Check sheet for the modelled part. Datum: model origin and axes. Units: mm. A direction names the side the tool comes from. Round coordinates to 2 decimals unless told otherwise and drop trailing zeros. Order: outer loops, then holes, each group sorted by start corner. A loop starts at its lowest first (then second) coordinate and runs counter-clockwise, first axis right, second up.
Autodesk Inventor part; units mm, degrees
ref_plane "a1_XY" through (0, 8.636, -14.224) normal (0, 1, 0) x (1, 0, 0)
ref_plane "a1_YZ" through (0, 8.636, -14.224) normal (1, 0, 0) x (0, 0, -1)
ref_plane "a1_ZX" through (0, 8.636, -14.224) normal (0, 0, -1) x (0, 1, 0)
sketch "Sketch_1" plane through (0, 0, 0) normal (0, 0, 1) x (1, 0, 0)
  line L0 (0, 0) -> (0, 8.636)
  line L1 (0, 8.636) -> (14.224, 8.636)
  line L2 (14.224, 8.636) -> (14.224, 0)
  line L3 (14.224, 0) -> (0, 0)
  line L4 (0, 0) -> (0, 8.636)
revolve "Revolution1" add sketch "Sketch_1" angle 360 about axis through (0, 0, 0) along (0, -1, 0)
sketch "Sketch_37" plane through (0, 0, 0) normal (0, 0, 1) x (1, 0, 0)
  line L0 (-5.9667, 5.08) -> (-14.224, 5.08)
  line L1 (-14.224, 5.08) -> (-14.224, 9.0488)
  line L2 (-14.224, 9.0488) -> (-13.716, 9.0488)
  line L3 (-13.716, 9.0488) -> (-13.716, 7.493)
  line L4 (-13.716, 7.493) -> (-13.2867, 7.0637)
  line L5 (-13.2867, 7.0637) -> (-7.112, 7.0637)
  line L6 (-7.112, 7.0637) -> (-5.9667, 5.08)
  line L7 (-5.9667, 5.08) -> (-14.224, 5.08)
revolve "Revolution2" cut sketch "Sketch_37" angle 360 about axis through (-5.9667, 5.08, 0) along (1, 0, 0)
thread "Thread1"
sketch "Sketch3" plane through (0, 0, 0) normal (0, -1, 0) x (1, 0, 0)
  point P0 (0, 0)
hole "Hole1" at (0, 0, 0) direction (0, 1, 0) diameter 15.494 depth 2.54
sketch "Sketch4" plane through (0, 8.636, 0) normal (0, 1, 0) x (1, 0, 0)
  point P0 (0, -11.176)
hole "Hole2" at (0, 8.636, 11.176) direction (0, -1, 0) diameter 3.048 depth 8.636 counterbore diameter 4.7752 counterbore depth 3.048
sketch "Sketch5" plane through (0, 8.636, 0) normal (0, 1, 0) x (1, 0, 0)
  point P0 (0, 11.176)
hole "Hole3" at (0, 8.636, -11.176) direction (0, -1, 0) diameter 3.048 depth 8.636 counterbore diameter 4.7752 counterbore depth 3.048
sketch "Sketch6" plane through (0, 0, 0) normal (0, -1, 0) x (1, 0, 0)
  point P0 (-7.9026, 7.9026)
hole "Hole4" at (-7.9026, 0, 7.9026) direction (0, 1, 0) diameter 3.048 depth 2.54
sketch "Sketch7" plane through (0, 0, 0) normal (0, -1, 0) x (1, 0, 0)
  point P0 (7.9026, 7.9026)
hole "Hole5" at (7.9026, 0, 7.9026) direction (0, 1, 0) diameter 3.048 depth 2.54
sketch "Sketch8" plane through (0, 0, 0) normal (0, -1, 0) x (1, 0, 0)
  point P0 (7.9026, -7.9026)
hole "Hole6" at (7.9026, 0, -7.9026) direction (0, 1, 0) diameter 3.048 depth 2.54
sketch "Sketch9" plane through (0, 0, 0) normal (0, -1, 0) x (1, 0, 0)
  point P0 (-7.9026, -7.9026)
hole "Hole7" at (-7.9026, 0, -7.9026) direction (0, 1, 0) diameter 3.048 depth 2.54
ref_plane "a1_XY" through (0, 8.636, -14.224) normal (0, 1, 0) x (1, 0, 0)
ref_plane "a1_YZ" through (0, 8.636, -14.224) normal (1, 0, 0) x (0, 0, -1)
ref_plane "a1_ZX" through (0, 8.636, -14.224) normal (0, 0, -1) x (0, 1, 0)
ref_plane "a2_XY" through (0, 8.636, 14.224) normal (0, 1, 0) x (1, 0, 0)
ref_plane "a2_YZ" through (0, 8.636, 14.224) normal (1, 0, 0) x (0, 0, -1)
ref_plane "a2_ZX" through (0, 8.636, 14.224) normal (0, 0, -1) x (0, 1, 0)
ref_plane "ar3_XY" through (-7.9026, 2.54, 7.9026) normal (0, 1, 0) x (1, 0, 0)
ref_plane "ar3_YZ" through (-7.9026, 2.54, 7.9026) normal (1, 0, 0) x (0, 0, -1)
ref_plane "ar3_ZX" through (-7.9026, 2.54, 7.9026) normal (0, 0, -1) x (0, 1, 0)
ref_plane "ar4_XY" through (7.9026, 2.54, 7.9026) normal (0, 1, 0) x (1, 0, 0)
ref_plane "ar4_YZ" through (7.9026, 2.54, 7.9026) normal (1, 0, 0) x (0, 0, -1)
ref_plane "ar4_ZX" through (7.9026, 2.54, 7.9026) normal (0, 0, -1) x (0, 1, 0)
ref_plane "ar5_XY" through (7.9026, 2.54, -7.9026) normal (0, 1, 0) x (1, 0, 0)
ref_plane "ar5_YZ" through (7.9026, 2.54, -7.9026) normal (1, 0, 0) x (0, 0, -1)
ref_plane "ar5_ZX" through (7.9026, 2.54, -7.9026) normal (0, 0, -1) x (0, 1, 0)
ref_plane "ar6_XY" through (-7.9026, 2.54, -7.9026) normal (0, 1, 0) x (1, 0, 0)
ref_plane "ar6_YZ" through (-7.9026, 2.54, -7.9026) normal (1, 0, 0) x (0, 0, -1)
ref_plane "ar6_ZX" through (-7.9026, 2.54, -7.9026) normal (0, 0, -1) x (0, 1, 0)
ref_plane "b1_XY" through (0, 8.636, 0) normal (0, 1, 0) x (1, 0, 0)
ref_plane "b1_YZ" through (0, 8.636, 0) normal (1, 0, 0) x (0, 0, -1)
ref_plane "b1_ZX" through (0, 8.636, 0) normal (0, 0, -1) x (0, 1, 0)
ref_plane "c1_XY" through (0, 8.636, -11.176) normal (0, 1, 0) x (1, 0, 0)
ref_plane "c1_YZ" through (0, 8.636, -11.176) normal (1, 0, 0) x (0, 0, -1)
ref_plane "c1_ZX" through (0, 8.636, -11.176) normal (0, 0, -1) x (0, 1, 0)
ref_plane "c2_XY" through (0, 8.636, 11.176) normal (0, 1, 0) x (1, 0, 0)
ref_plane "c2_YZ" through (0, 8.636, 11.176) normal (1, 0, 0) x (0, 0, -1)
ref_plane "c2_ZX" through (0, 8.636, 11.176) normal (0, 0, -1) x (0, 1, 0)
ref_plane "d1_XY" through (-1.524, 8.636, -11.176) normal (0, 1, 0) x (1, 0, 0)
ref_plane "d1_YZ" through (-1.524, 8.636, -11.176) normal (1, 0, 0) x (0, 0, -1)
ref_plane "d1_ZX" through (-1.524, 8.636, -11.176) normal (0, 0, -1) x (0, 1, 0)
ref_plane "d2_XY" through (1.524, 8.636, -11.176) normal (0, 1, 0) x (1, 0, 0)
ref_plane "d2_YZ" through (1.524, 8.636, -11.176) normal (1, 0, 0) x (0, 0, -1)
ref_plane "d2_ZX" through (1.524, 8.636, -11.176) normal (0, 0, -1) x (0, 1, 0)
ref_plane "j_XY" through (0, 0, 0) normal (0, 1, 0) x (1, 0, 0)
ref_plane "j_YZ" through (0, 0, 0) normal (1, 0, 0) x (0, 0, -1)
ref_plane "j_ZX" through (0, 0, 0) normal (0, 0, -1) x (0, 1, 0)
ref_plane "k1_XY" through (-14.224, 5.08, 0) normal (0, 0, 1) x (1, 0, 0)
ref_plane "k1_YZ" through (-14.224, 5.08, 0) normal (1, 0, 0) x (0, 1, 0)
ref_plane "k1_ZX" through (-14.224, 5.08, 0) normal (0, 1, 0) x (0, 0, 1)
ref_plane "k2_XY" through (-14.224, 8.636, 0) normal (0, 0, 1) x (1, 0, 0)
ref_plane "k2_YZ" through (-14.224, 8.636, 0) normal (1, 0, 0) x (0, 1, 0)
ref_plane "k2_ZX" through (-14.224, 8.636, 0) normal (0, 1, 0) x (0, 0, 1)
ref_plane "l1_XY" through (-14.224, 7.493, 0) normal (0, 0, 1) x (1, 0, 0)
ref_plane "l1_YZ" through (-14.224, 7.493, 0) normal (1, 0, 0) x (0, 1, 0)
ref_plane "l1_ZX" through (-14.224, 7.493, 0) normal (0, 1, 0) x (0, 0, 1)
ref_plane "l2_XY" through (-14.224, 2.667, 0) normal (0, 0, 1) x (1, 0, 0)
ref_plane "l2_YZ" through (-14.224, 2.667, 0) normal (1, 0, 0) x (0, 1, 0)
ref_plane "l2_ZX" through (-14.224, 2.667, 0) normal (0, 1, 0) x (0, 0, 1)
ref_plane "rg_XY" through (0, 8.636, 0) normal (0, 1, 0) x (1, 0, 0)
ref_plane "rg_YZ" through (0, 8.636, 0) normal (1, 0, 0) x (0, 0, -1)
ref_plane "rg_ZX" through (0, 8.636, 0) normal (0, 0, -1) x (0, 1, 0)
ref_plane "rh_XY" through (0, 8.636, 0) normal (0, 1, 0) x (1, 0, 0)
ref_plane "rh_YZ" through (0, 8.636, 0) normal (1, 0, 0) x (0, 0, -1)
ref_plane "rh_ZX" through (0, 8.636, 0) normal (0, 0, -1) x (0, 1, 0)
ref_plane "to_dummy_XY" through (0, 8.636, 0) normal (0, 1, 0) x (1, 0, 0)
ref_plane "to_dummy_YZ" through (0, 8.636, 0) normal (1, 0, 0) x (0, 0, -1)
ref_plane "to_dummy_ZX" through (0, 8.636, 0) normal (0, 0, -1) x (0, 1, 0)
ref_plane "to_nut_XY" through (0, 10.16, 0) normal (0, 1, 0) x (1, 0, 0)
ref_plane "to_nut_YZ" through (0, 10.16, 0) normal (1, 0, 0) x (0, 0, -1)
ref_plane "to_nut_ZX" through (0, 10.16, 0) normal (0, 0, -1) x (0, 1, 0)
ref_plane "to_rod_XY" through (0, 8.636, 0) normal (0, 1, 0) x (1, 0, 0)
ref_plane "to_rod_YZ" through (0, 8.636, 0) normal (1, 0, 0) x (0, 0, -1)
ref_plane "to_rod_ZX" through (0, 8.636, 0) normal (0, 0, -1) x (0, 1, 0)
ref_plane "to_tube_XY" through (0, 2.54, 0) normal (0, 1, 0) x (1, 0, 0)
ref_plane "to_tube_YZ" through (0, 2.54, 0) normal (1, 0, 0) x (0, 0, -1)
ref_plane "to_tube_ZX" through (0, 2.54, 0) normal (0, 0, -1) x (0, 1, 0)
ref_plane "to_wiper_XY" through (0, 8.636, 0) normal (0, 1, 0) x (1, 0, 0)
ref_plane "to_wiper_YZ" through (0, 8.636, 0) normal (1, 0, 0) x (0, 0, -1)
ref_plane "to_wiper_ZX" through (0, 8.636, 0) normal (0, 0, -1) x (0, 1, 0)
ref_plane "track1_XY" through (-7.874, 0, 0) normal (0, 1, 0) x (1, 0, 0)
ref_plane "track1_YZ" through (-7.874, 0, 0) normal (1, 0, 0) x (0, 0, -1)
ref_plane "track1_ZX" through (-7.874, 0, 0) normal (0, 0, -1) x (0, 1, 0)
ref_plane "track2_XY" through (0, 0, -7.874) normal (0, 1, 0) x (1, 0, 0)
ref_plane "track2_YZ" through (0, 0, -7.874) normal (1, 0, 0) x (0, 0, -1)
ref_plane "track2_ZX" through (0, 0, -7.874) normal (0, 0, -1) x (0, 1, 0)
ref_plane "track3_XY" through (7.874, 0, 0) normal (0, 1, 0) x (1, 0, 0)
ref_plane "track3_YZ" through (7.874, 0, 0) normal (1, 0, 0) x (0, 0, -1)
ref_plane "track3_ZX" through (7.874, 0, 0) normal (0, 0, -1) x (0, 1, 0)
ref_plane "track4_XY" through (0, 0, 7.874) normal (0, 1, 0) x (1, 0, 0)
ref_plane "track4_YZ" through (0, 0, 7.874) normal (1, 0, 0) x (0, 0, -1)
ref_plane "track4_ZX" through (0, 0, 7.874) normal (0, 0, -1) x (0, 1, 0)
properties part number "02-2-0.13-FO1_BM_heads" material "Steel"
Item 1: Sectioned sample at A-A (x = 0). Record the cut outline in (y, z), and give its area (3 significant figures).
Answer:
outline: (0, -14.22) - (8.64, -14.22) - (8.64, -13.56) - (5.59, -13.56) - (5.59, -12.7) - (0, -12.7) - close; (0, -9.65) - (5.59, -9.65) - (5.59, -8.79) - (8.64, -8.79) - (8.64, 8.79) - (5.59, 8.79) - (5.59, 9.65) - (0, 9.65) - (0, 7.75) - (2.54, 7.75) - (2.54, -7.75) - (0, -7.75) - close; (0, 12.7) - (5.59, 12.7) - (5.59, 13.56) - (8.64, 13.56) - (8.64, 14.22) - (0, 14.22) - close
area: 143 mm2
Item 2: Sectioned sample at C-C (y = 8). Record the cut outline in (x, z).
Answer:
outline: (-13.97, -2.69) arc R14.22 ccw (long way) to (-13.97, 2.69) - (-13.72, 2.69) - (-13.72, -2.69) - close; hole circle Ø4.78 at (0, -11.18); hole circle Ø4.78 at (0, 11.18)
Item 3: Go/stop test with flat-tipped pins: P1, Ø2.5, axis at x = 7.9, z = -7.9, coming from the -Y side; P2, Ø3, axis at y = 5.08, z = 0, coming from the -X side; P3, Ø3, axis at y = 6.5, z = 8, coming from the -X side; P4, Ø1.8, axis at x = 0, z = -11.176, coming from the +Y side. Record where each tip stops, or that it passes through.
Answer:
P1: stops at y = 2.54
P2: stops at x = -6.83
P3: stops at x = -12.65
P4: passes through
Item 4: Sectioned sample at B-B (x = -11). Record the cut outline in (y, z).
Answer:
outline: (0, -9.02) - (8.64, -9.02) - (8.64, 9.02) - (0, 9.02) - close; hole circle Ø3.97 at (5.08, 0)
Item 5: Release check for a two-part mould opening along Y. For faces 1 (the conical face through (-6.166, 4.736, -0.015)), 2 (the flat face through (6, 0, -6)), 3 (the cylindrical face through (8.49, 1.29, -9.31)) record: released by +Y, released by -Y, zero draft, split by the parting line, or undercut.
Answer:
face 1: undercut
face 2: released by -Y
face 3: zero draft
Item 6: Sectioned sample at D-D (z = -5.5). Record the cut outline in (x, y).
Answer:
outline: (-13.12, 0) - (-5.46, 0) - (-5.46, 2.54) - (5.46, 2.54) - (5.46, 0) - (13.12, 0) - (13.12, 8.64) - (-13.12, 8.64) - close
Item 7: Access from +Z, -Z, +X, -X, +Y, -Y to the whole of each face (thin tool, end or side, straight path). Record for faces 4 (the cylindrical face through (-13.91, 1.11, 0.07)), 5 (the flat face through (8, 2.54, -8)), 6 (the cylindrical face through (-0.1, 7.09, -13.56)).
Answer:
face 4: -X
face 5: -Y
face 6: +Y
Item 8: Scan lines: line 1 along Z through (x, y) = (0, 7.6); line 2 along Z through (x, y) = (0, 3.75); line 3 along Z through (x, y) = (-0.75, 1.75). Record each from-to range of solid material in increasing order.
Answer:
line 1: z = -14.22 to -13.56, -8.79 to 8.79, 13.56 to 14.22
line 2: z = -14.22 to -12.7, -9.65 to 9.65, 12.7 to 14.22
line 3: z = -14.2 to -12.5, -9.85 to -7.71, 7.71 to 9.85, 12.5 to 14.2
